Source: CAD feature listing. Evaluate the final solid. Frame: model axes, mm. A direction names the side the tool comes from. Give positions to 0.01 mm unless a question says otherwise; leave off trailing zeros. Write each loop counter-clockwise with the first axis right and the second up, starting at its lowest first coordinate (ties: lowest second). Pieces come first, ordered by that corner, then holes. Notation, with made-up numbers: (87.5, 67.5) -> (128.5, 67.5) arc R37 cw to (128.5, 106.5) -> close; hole circle Ø11 at (-26, 24.25). An arc over 180 degrees is marked (long way). Write item = value, one per line.
from build123d import *

# Parameters (mm, degrees)
F0_R          = 41
F1_DEPTH      = 3
F1_TAPER      = -45
F2_R          = 32.5
F3_DEPTH      = 10
F4_W          = 10
F4_H          = 6
F6_DEPTH      = 33
F6_DEPTH_BACK = 33
F7_W          = 10
F7_H          = 6
F8_DEPTH      = 33
F8_DEPTH_BACK = 33
F5_R          = 30.5
F9_DEPTH      = 7
F12_DEPTH     = 7
F13_SIZE2     = 2
F13_SIZE      = 3
F13_2_SIZE2   = 2
F13_2_SIZE    = 3
F14_SIZE2     = 3
F14_SIZE      = 2
F14_2_SIZE2   = 3
F14_2_SIZE    = 2
F15_T4_DEPTH  = 20.3593154951
F15_S5_R      = 32.5
F15_T6_DEPTH  = 12
F15_T10_DEPTH = 20.3593154951
F15_S11_R     = 32.5
F15_T12_DEPTH = 12
F16_T4_DEPTH  = 20.3593154951
F16_S5_R      = 32.5
F16_T6_DEPTH  = 12
F16_T10_DEPTH = 20.3593154951
F16_S11_R     = 32.5
F16_T12_DEPTH = 12


# Not quite as in the source:
# - a fillet or chamfer that OpenCascade refuses, or shapes differently, is made with other operations: its cross-section is extruded or revolved along the edge and cut away or added


with BuildPart() as f1:
    # F0 (on Top) → F1 (new body)
    with BuildSketch(Plane.XY):
        Circle(F0_R)
    extrude(amount=F1_DEPTH, taper=F1_TAPER)

    # F2 (on face) → F3 (join)
    with BuildSketch(Plane.XY.offset(3)):
        Circle(F2_R)
    extrude(amount=F3_DEPTH)

    # F4 (on Front) → F6 (join, two sides)
    with BuildSketch(Plane.XZ) as f6_sk:
        with Locations((0, 10)):
            Rectangle(F4_W, F4_H)
    extrude(amount=F6_DEPTH)
    extrude(f6_sk.sketch, amount=-F6_DEPTH_BACK)

    # F7 (on Right) → F8 (join, two sides)
    with BuildSketch(Plane.YZ) as f8_sk:
        with Locations((0, 10)):
            Rectangle(F7_W, F7_H)
    extrude(amount=F8_DEPTH)
    extrude(f8_sk.sketch, amount=-F8_DEPTH_BACK)

    # F5 (on face) → F9 (cut)
    with BuildSketch(Plane.XY.offset(13)):
        Circle(F5_R)
    extrude(amount=-F9_DEPTH, mode=Mode.SUBTRACT)

    # F11 (on face) → F12 (cut)
    with BuildSketch(Plane.XY.offset(13)):
        with BuildLine():
            ThreePointArc((-5.6789083458, 32), (-22.9809703886, 22.9809703886), (-32, 5.6789083458))
            Line((-32, 5.6789083458), (-29.9666481275, 5.6789083458))
            ThreePointArc((-29.9666481275, 5.6789083458), (-21.5667568262, 21.5667568262), (-5.6789083458, 29.9666481275))
            Line((-5.6789083458, 29.9666481275), (-5.6789083458, 32))
        make_face()
        with BuildLine():
            ThreePointArc((-5.6789083458, 29.9666481275), (-21.5667568262, 21.5667568262), (-29.9666481275, 5.6789083458))
            ThreePointArc((-29.9666481275, 5.6789083458), (-30.5, 0), (-29.9666481275, -5.6789083458))
            ThreePointArc((-29.9666481275, -5.6789083458), (-21.5667568262, -21.5667568262), (-5.6789083458, -29.9666481275))
            ThreePointArc((-5.6789083458, -29.9666481275), (0, -30.5), (5.6789083458, -29.9666481275))
            ThreePointArc((5.6789083458, -29.9666481275), (21.5667568262, -21.5667568262), (29.9666481275, -5.6789083458))
            ThreePointArc((29.9666481275, -5.6789083458), (30.3663692915, -2.8519495183), (30.5, 0))
            ThreePointArc((30.5, 0), (30.3663692915, 2.8519495183), (29.9666481275, 5.6789083458))
            ThreePointArc((29.9666481275, 5.6789083458), (21.5667568262, 21.5667568262), (5.6789083458, 29.9666481275))
            ThreePointArc((5.6789083458, 29.9666481275), (0, 30.5), (-5.6789083458, 29.9666481275))
        make_face()
        with BuildLine():
            Line((5.6789083458, 32), (5.6789083458, 29.9666481275))
            ThreePointArc((5.6789083458, 29.9666481275), (21.5667568262, 21.5667568262), (29.9666481275, 5.6789083458))
            Line((29.9666481275, 5.6789083458), (32, 5.6789083458))
            ThreePointArc((32, 5.6789083458), (22.9809703886, 22.9809703886), (5.6789083458, 32))
        make_face()
        with BuildLine():
            ThreePointArc((29.9666481275, -5.6789083458), (21.5667568262, -21.5667568262), (5.6789083458, -29.9666481275))
            Line((5.6789083458, -29.9666481275), (5.6789083458, -32))
            ThreePointArc((5.6789083458, -32), (22.9809703886, -22.9809703886), (32, -5.6789083458))
            Line((32, -5.6789083458), (29.9666481275, -5.6789083458))
        make_face()
        with BuildLine():
            ThreePointArc((-5.6789083458, -29.9666481275), (-21.5667568262, -21.5667568262), (-29.9666481275, -5.6789083458))
            Line((-29.9666481275, -5.6789083458), (-32, -5.6789083458))
            ThreePointArc((-32, -5.6789083458), (-22.9809703886, -22.9809703886), (-5.6789083458, -32))
            Line((-5.6789083458, -32), (-5.6789083458, -29.9666481275))
        make_face()
    extrude(amount=-F12_DEPTH, mode=Mode.SUBTRACT)

    # F13
    f13_edges = [f1.edges().sort_by_distance(p)[0] for p in [
        (0, 33, 13),
    ]]
    f13_side = f1.faces().sort_by_distance((0, 33, 10))[0]
    chamfer(f13_edges, length=F13_SIZE, length2=F13_SIZE2, reference=f13_side)

    # F13#2
    f13_2_edges = [f1.edges().sort_by_distance(p)[0] for p in [
        (33, 0, 13),
    ]]
    f13_2_side = f1.faces().sort_by_distance((33, 0, 10))[0]
    chamfer(f13_2_edges, length=F13_2_SIZE, length2=F13_2_SIZE2, reference=f13_2_side)

    # F14
    f14_edges = [f1.edges().sort_by_distance(p)[0] for p in [
        (0, -33, 13),
    ]]
    f14_side = f1.faces().sort_by_distance((0, -31.618427, 13))[0]
    chamfer(f14_edges, length=F14_SIZE, length2=F14_SIZE2, reference=f14_side)

    # F14#2
    f14_2_edges = [f1.edges().sort_by_distance(p)[0] for p in [
        (-33, 0, 13),
    ]]
    f14_2_side = f1.faces().sort_by_distance((-31.618427, 0, 13))[0]
    chamfer(f14_2_edges, length=F14_2_SIZE, length2=F14_2_SIZE2, reference=f14_2_side)

    # F15: chamfer of 1 x 2 on 2 edges, made by hand


with BuildPart() as f15_tool2:
    # F15_s3 → F15_t4 (new body)
    with BuildSketch(Plane.XZ.offset(10.1796577476)):
        Polygon((32, 7), (33, 9), (33, 7), align=None)
    extrude(amount=-F15_T4_DEPTH)

    # F15_s5 → F15_t6 (cut, symmetric)
    with BuildSketch(Plane.XY.offset(8)):
        Circle(F15_S5_R)
    extrude(amount=F15_T6_DEPTH, both=True, mode=Mode.SUBTRACT)


with BuildPart() as f1_1:
    add(f1.part)

    # F15_t1: cut F15_tool2
    add(f15_tool2.part, mode=Mode.SUBTRACT)


with BuildPart() as f15_tool8:
    # F15_s9 → F15_t10 (new body)
    with BuildSketch(Plane.YZ.offset(-10.1796577476)):
        Polygon((32, 7), (33, 9), (33, 7), align=None)
    extrude(amount=F15_T10_DEPTH)

    # F15_s11 → F15_t12 (cut, symmetric)
    with BuildSketch(Plane.XY.offset(8)):
        Circle(F15_S11_R)
    extrude(amount=F15_T12_DEPTH, both=True, mode=Mode.SUBTRACT)


with BuildPart() as f1_2:
    add(f1_1.part)

    # F15_t7: cut F15_tool8
    add(f15_tool8.part, mode=Mode.SUBTRACT)

    # F16: chamfer of 2 x 1 on 2 edges, made by hand


with BuildPart() as f16_tool2:
    # F16_s3 → F16_t4 (new body)
    with BuildSketch(Plane.YZ.offset(-10.1796577476)):
        Polygon((-33, 9), (-32, 7), (-33, 7), align=None)
    extrude(amount=F16_T4_DEPTH)

    # F16_s5 → F16_t6 (cut, symmetric)
    with BuildSketch(Plane.XY.offset(8)):
        Circle(F16_S5_R)
    extrude(amount=F16_T6_DEPTH, both=True, mode=Mode.SUBTRACT)


with BuildPart() as f1_3:
    add(f1_2.part)

    # F16_t1: cut F16_tool2
    add(f16_tool2.part, mode=Mode.SUBTRACT)


with BuildPart() as f16_tool8:
    # F16_s9 → F16_t10 (new body)
    with BuildSketch(Plane.XZ.offset(10.1796577476)):
        Polygon((-33, 9), (-32, 7), (-33, 7), align=None)
    extrude(amount=-F16_T10_DEPTH)

    # F16_s11 → F16_t12 (cut, symmetric)
    with BuildSketch(Plane.XY.offset(8)):
        Circle(F16_S11_R)
    extrude(amount=F16_T12_DEPTH, both=True, mode=Mode.SUBTRACT)


with BuildPart() as f1_4:
    add(f1_3.part)

    # F16_t7: cut F16_tool8
    add(f16_tool8.part, mode=Mode.SUBTRACT)


solid = f1_4.part
1) Cut plane B-B (z = 1.25). Return the cut outline in (x, y).
Computed:
outline = circle Ø84.5 at (0, 0)
2) Cut plane A-A (x = 0). Return the cut outline in (y, z), then the cut area to 4 significant figures.
Computed:
outline = (-44, 3) -> (-41, 0) -> (41, 0) -> (44, 3) -> (32.5, 3) -> (32.5, 8) -> (33, 9) -> (33, 10) -> (31, 13) -> (30.5, 13) -> (30.5, 6) -> (-30.5, 6) -> (-30.5, 13) -> (-31, 13) -> (-33, 10) -> (-33, 9) -> (-32.5, 8) -> (-32.5, 3) -> close
area = 476.5 mm²
3) Material intervals for L1, parallel to Z at x = -38, y = 8.5; L2, parallel to Z at x = -5, y = 12; L3, parallel to Y at x = -4, z = 7, sorted ascending.
Computed:
L1 = 0 to 3
L2 = 0 to 6
L3 = -32.25 to -30.24, 30.24 to 32.25
4) Contact query for flat-ended pins moving along their axis: pin 1 (2 mm diameter, centred on x = 31, z = 8, fed in from +Y); pin 2 (0.6 mm diameter, centred on y = 31, z = 10, fed in from +X); pin 3 (6 mm diameter, centred on y = 16.5, z = 5.5, fed in from -X). Output: stop coordinate, or through.
Computed:
pin_1 = 5.68
pin_2 = 5.68
pin_3 = -41.42
5) Access query for faces 1 (the cylindrical face through (0.1, 30.5, 9.5)), 2 (the flat face through (31, -5.679, 10)), 3 (the flat face through (5.679, -31, 10)), 4 (the flat face through (-5.679, 31, 10)), 5 (the flat face through (-31, 5.679, 10)). Directions: +Z, -Z, +X, -X, +Y, -Y. A direction counts if a zero-diameter tool reaches every point of the face in a straight line with its end or side. Return the directions, or none.
Computed:
face_1 = +Z
face_2 = +Z, +X, -X, -Y
face_3 = +Z, +X, +Y, -Y
face_4 = +Z, -X, +Y, -Y
face_5 = +Z, +X, -X, +Y
